from build123d import *

# Parameters (mm, degrees)
EXTRUDE_1_DEPTH          = 400
CUT_EXTRUDE_2_DEPTH      = 401.140600289
CUT_EXTRUDE_2_DEPTH_BACK = 401.140600289
SKETCH_2_4_R             = 1.65


with BuildPart() as part:
    # Sketch 2 → Extrude 1 (new body)
    with BuildSketch(Plane(origin=(0, 0, 0), x_dir=(0, 0, -1), z_dir=(1, 0, 0))):
        with BuildLine():
            Line((-7, 7.5), (7, 7.5))
            ThreePointArc((7, 7.5), (7.353553391, 7.353553391), (7.5, 7))
            Line((7.5, 7), (7.5, -7))
            ThreePointArc((7.5, -7), (7.353553391, -7.353553391), (7, -7.5))
            Line((7, -7.5), (-7, -7.5))
            ThreePointArc((-7, -7.5), (-7.353553391, -7.353553391), (-7.5, -7))
            Line((-7.5, -7), (-7.5, 7))
            ThreePointArc((-7.5, 7), (-7.353553391, 7.353553391), (-7, 7.5))
        make_face()
    extrude(amount=EXTRUDE_1_DEPTH)

    # Sketch 2_4 → Cut-Extrude 2 (cut, two sides: drawn at the far end of the back side and taken through both)
    with BuildSketch(Plane(origin=(0, 0, 0), x_dir=(0, 0, -1), z_dir=(1, 0, 0)).offset(-CUT_EXTRUDE_2_DEPTH_BACK)):
        Polygon((-3.1, -6.5), (-3.1, -7.5), (3.1, -7.5), (3.1, -6.5), (4.7, -6.5), (4.7, -5.407106781), (2.092893219, -2.8), (-2.092893219, -2.8), (-4.7, -5.407106781), (-4.7, -6.5), align=None)
        Polygon((-6.5, 3.1), (-7.5, 3.1), (-7.5, -3.1), (-6.5, -3.1), (-6.5, -4.7), (-5.407106781, -4.7), (-2.8, -2.092893219), (-2.8, 2.092893219), (-5.407106781, 4.7), (-6.5, 4.7), align=None)
        Polygon((4.7, 6.5), (3.1, 6.5), (3.1, 7.5), (-3.1, 7.5), (-3.1, 6.5), (-4.7, 6.5), (-4.7, 5.407106781), (-2.092893219, 2.8), (2.092893219, 2.8), (4.7, 5.407106781), align=None)
        Polygon((7.5, -3.1), (7.5, 3.1), (6.5, 3.1), (6.5, 4.7), (5.407106781, 4.7), (2.8, 2.092893219), (2.8, -2.092893219), (5.407106781, -4.7), (6.5, -4.7), (6.5, -3.1), align=None)
        Circle(SKETCH_2_4_R)
    extrude(amount=CUT_EXTRUDE_2_DEPTH + CUT_EXTRUDE_2_DEPTH_BACK, mode=Mode.SUBTRACT)


solid = part.part
The listing builds one solid part. Answer for the finished solid, in the listing's coordinates (mm). Coordinates: 2 decimals unless noted, no trailing zeros.
Q1. Given P1, Ø1.3, axis at x = 130.5, z = -0.5, coming from the +Y side; P2, Ø1.5, axis at x = 113, y = 2, coming from the -Z side; P3, Ø1.5, axis at x = 250.5, y = 0, coming from the -Z side; P4, Ø3, axis at y = 1.5, z = 4.5, coming from the -X side, each flat-ended and moving along its own axis, determine where each tip first touches the part or whether it passes through.
Q2. Consider line 1 (Y direction, x = 315, z = 0); line 2 (Z direction, x = 335, y = -0.25); line 3 (Z direction, x = 120.5, y = -4). Determine where each line is inside the solid, lowest interval first.
Q3. For a pull along X with two mould halves and no side action, classify faces 1 (the face through (400, 2, 0)), 2 (the face through (0, 2, 0)) as pulls with the +X half, pulls with the -X half, needs draft (parallel to the pull), parting line crosses it, or undercut.
Answers follow:
1. P1: stops at y = 2.8
1. P2: stops at z = -3.46
1. P3: stops at z = -2.8
1. P4: passes through
2. line 1: y = -2.8 to -1.65, 1.65 to 2.8
2. line 2: z = -2.8 to -1.63, 1.63 to 2.8
2. line 3: z = -7.5 to -6.5, -4.71 to -3.29, 3.29 to 4.71, 6.5 to 7.5
3. face 1: pulls with the +X half
3. face 2: pulls with the -X half
